from build123d import *

# Parameters (mm, degrees)
F1_DEPTH       = 25
F2_R           = 5
F3_R           = 5
F5_D           = 4.4958
F5_DEPTH       = 5
F5_CSINK_D     = 9.1186
F5_CSINK_ANGLE = 82
F5_TIP         = 1.3506745855


with BuildPart() as f1:
    # F0 (on Top) → F1 (new body)
    with BuildSketch(Plane.XY):
        with BuildLine():
            ThreePointArc((65.5, -63), (54.4714923246, -26.6254687462), (25.099800796, -2.5))
            Line((25.099800796, -2.5), (11.0453610172, -2.5))
            ThreePointArc((11.0453610172, -2.5), (47.2310263627, -23.6111672079), (61.5, -63))
            ThreePointArc((61.5, -63), (-39.3888327921, -110.2310263627), (-11.0453610172, -2.5))
            Line((-11.0453610172, -2.5), (-25.099800796, -2.5))
            ThreePointArc((-25.099800796, -2.5), (-36.3745312538, -117.4714923246), (65.5, -63))
        make_face()
        with BuildLine():
            Line((0, 2.5), (-100.5, 2.5))
            Line((-100.5, 2.5), (-100.5, -2.5))
            Line((-100.5, -2.5), (-25.099800796, -2.5))
            ThreePointArc((-25.099800796, -2.5), (-12.7964838921, 1.2378393161), (0, 2.5))
        make_face()
        with BuildLine():
            ThreePointArc((25.099800796, -2.5), (12.7964838921, 1.2378393161), (0, 2.5))
            ThreePointArc((0, 2.5), (-12.7964838921, 1.2378393161), (-25.099800796, -2.5))
            Line((-25.099800796, -2.5), (-11.0453610172, -2.5))
            ThreePointArc((-11.0453610172, -2.5), (0, -1.5), (11.0453610172, -2.5))
            Line((11.0453610172, -2.5), (25.099800796, -2.5))
        make_face()
        with BuildLine():
            Line((100.5, 2.5), (0, 2.5))
            ThreePointArc((0, 2.5), (12.7964838921, 1.2378393161), (25.099800796, -2.5))
            Line((25.099800796, -2.5), (100.5, -2.5))
            Line((100.5, -2.5), (100.5, 2.5))
        make_face()
    extrude(amount=F1_DEPTH)

    # F2
    f2_edges = [f1.edges().sort_by_distance(p)[0] for p in [
        (-25.099801, -2.5, 12.5),
        (25.099801, -2.5, 12.5),
    ]]
    fillet(f2_edges, radius=F2_R)

    # F3
    f3_edges = [f1.edges().sort_by_distance(p)[0] for p in [
        (-100.5, 0, 25),
        (-100.5, 0, 0),
        (100.5, 0, 25),
        (100.5, 0, 0),
    ]]
    fillet(f3_edges, radius=F3_R)

    # F5
    with Locations(Plane.XZ.offset(2.5)):
        with Locations((-85.5, 12.5), (85.5, 12.5)):
            CounterSinkHole(F5_D / 2, F5_CSINK_D / 2, depth=F5_DEPTH, counter_sink_angle=F5_CSINK_ANGLE)
            with Locations((0, 0, -(F5_DEPTH + F5_TIP / 2))):  # 118° drill point
                Cone(0, F5_D / 2, F5_TIP, mode=Mode.SUBTRACT)


solid = f1.part
The listing builds one solid part. Answer for the finished solid, in the listing's coordinates (mm). A direction names the side the tool comes from. Round coordinates to 2 decimals unless told otherwise and drop trailing zeros. Write each loop counter-clockwise with the first axis right and the second up, starting at its lowest first coordinate (ties: lowest second). Pieces come first, ordered by that corner, then holes. Notation, with made-up numbers: M -33,36 L 15,36 A12 cw 15,54 Z; hole C 86,24 d3. An arc over 180 degrees is marked long. Write each question's results on one line, items separated by ' | '. Start each with the question number.
Item 1: Given pin 1 Ø7.5 at (x, z) = (73, 13.5) entering from -Y; pin 2 Ø6 at (y, z) = (-38.5, 10) entering from +X; pin 3 Ø1 at (y, z) = (-18, 4) entering from -X, each flat-ended and moving along its own axis, determine where each tip first touches the part or whether it passes through.
Item 2: Find section C-C on x = -47.5. Write down the section's boundary in (y, z).
Item 3: The mould has two halves that part along X. Classify faces 1 (the cylindrical face through (87.28, 1.35, 11.13)), 2 (the cylindrical face through (-99, -0.04, 23.57)), 3 (the cylindrical face through (99, 0.04, 1.43)), 4 (the conical face through (-83.14, 0.03, 12.6)): +X half, -X half, draft (parallel to the pull), parting line (faces both ways), or undercut.
Item 4: Straight lines are drawn through the part: probe 1 along X at (y, z) = (1.7, 12.5); probe 2 along Y at (x, z) = (-45.5, 16.5); probe 3 along Z at (x, y) = (85.5, 1.3). For each, find the intervals that lie inside material, in ascending order.
Item 5: Which of the six approach directions +Z, -Z, +X, -X, +Y, -Y give full straight-line access (tool end or side, diameter ignored) to faces 5 (the flat face through (100.5, 0, 12)), 6 (the flat face through (-72, -2.5, 12)), 7 (the flat face through (72, -2.5, 12))?
Item 6: Find section A-A on x = 0. Write down the section's boundary in (y, z).
Item 7: Find section D-D on x = -85.5. Write down the section's boundary in (y, z).
Item 8: Find section B-B on y = -95. Write down the section's boundary in (x, z).
Answer block:
1) pin 1: stops at y = -2.5 | pin 2: stops at x = 61.87 | pin 3: stops at x = -48.06
2) outline: M -108.1,0 L -102.06,0 L -102.06,25 L -108.1,25 Z; M -23.94,0 L -17.9,0 L -17.9,25 L -23.94,25 Z; M -2.5,0 L 2.5,0 L 2.5,25 L -2.5,25 Z
3) face 1: undercut | face 2: -X half | face 3: +X half | face 4: undercut
4) probe 1: x = -100.5 to -87.75, -83.25 to 83.25, 87.75 to 100.5 | probe 2: y = -110.12 to -104.38, -21.62 to -15.88, -2.5 to 2.5 | probe 3: z = 0 to 10.25, 14.75 to 25
5) face 5: +Z, -Z, +X, +Y, -Y | face 6: +Z, -Z, -X | face 7: +Z, -Z, +X
6) outline: M -128.5,0 L -124.5,0 L -124.5,25 L -128.5,25 Z; M -1.5,0 L 2.5,0 L 2.5,25 L -1.5,25 Z
7) outline: M -2.5,0 L 2.5,0 L 2.5,10.25 L 0.16,10.25 L -2.5,7.94 Z; M -2.5,17.06 L 0.16,14.75 L 2.5,14.75 L 2.5,25 L -2.5,25 Z
8) outline: M -57.15,0 L -52.52,0 L -52.52,25 L -57.15,25 Z; M 52.52,0 L 57.15,0 L 57.15,25 L 52.52,25 Z
